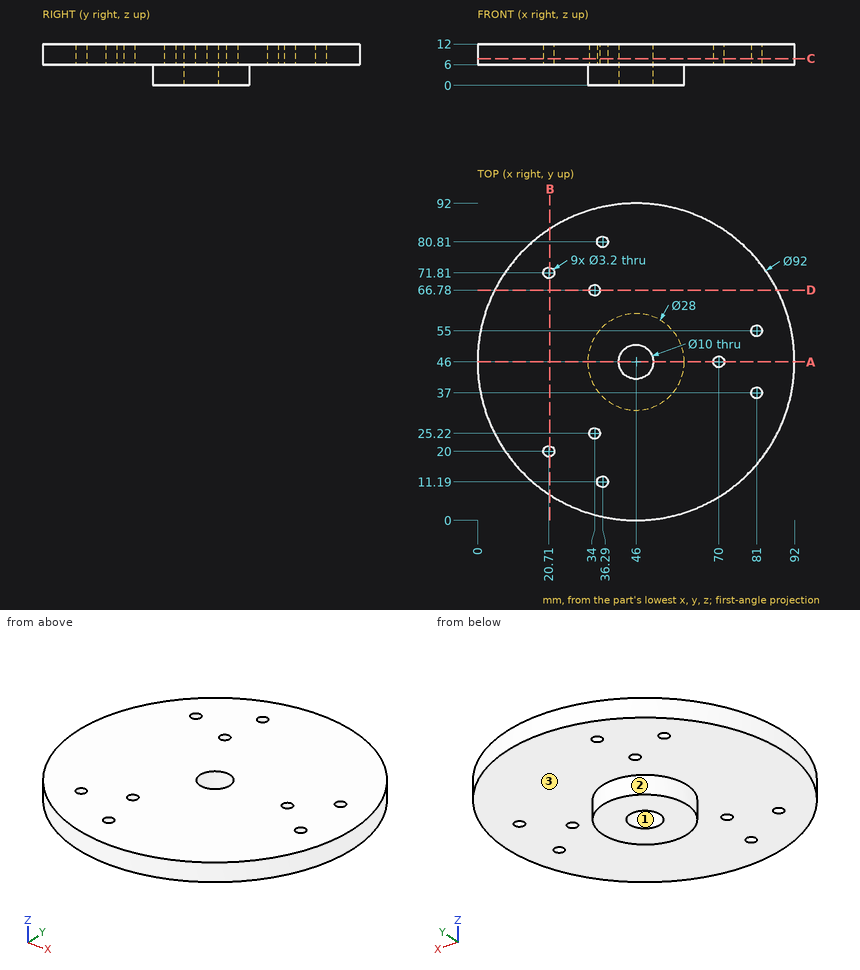
Study the drawing (mm; zero at the part's minimum x, y, z) and answer. Coordinates: 2 decimals unless noted, no trailing zeros. Write each loop counter-clockwise with the first axis right and the second up, starting at its lowest first coordinate (ties: lowest second). Pieces come first, ordered by that corner, then holes.
Q1. Find the intervals of material crossed by line 1 along Y through (x, z) = (36.29, 9.95); line 2 along Y through (x, z) = (81, 7.2); line 3 along Z through (x, y) = (45.5, 20.5), in increasing order.
Returned:
line 1: y = 1.04 to 9.59, 12.79 to 79.21, 82.41 to 90.96
line 2: y = 16.15 to 35.4, 38.6 to 53.4, 56.6 to 75.85
line 3: z = 6 to 12
Q2. Section D-D, the plane y = 66.78 is taken. Write down the section's boundary in (x, z).
Returned:
outline: (4.96, 6) - (32.4, 6) - (32.4, 12) - (4.96, 12) - close; (35.6, 6) - (87.04, 6) - (87.04, 12) - (35.6, 12) - close
Q3. Section B-B, the plane x = 21 is taken. Write down the section's boundary in (y, z).
Returned:
outline: (7.39, 6) - (18.43, 6) - (18.43, 12) - (7.39, 12) - close; (21.57, 6) - (70.24, 6) - (70.24, 12) - (21.57, 12) - close; (73.38, 6) - (84.61, 6) - (84.61, 12) - (73.38, 12) - close
Q4. Section A-A, the plane y = 46 is taken. Write down the section's boundary in (x, z), then the cut area to 3 significant figures.
Returned:
outline: (0, 6) - (32, 6) - (32, 0) - (41, 0) - (41, 12) - (0, 12) - close; (51, 0) - (60, 0) - (60, 6) - (68.4, 6) - (68.4, 12) - (51, 12) - close; (71.6, 6) - (92, 6) - (92, 12) - (71.6, 12) - close
area: 581 mm2
Q5. Given P1, Ø10, axis at x = 34, y = 25.5, coming from the -Z side; P2, Ø4, axis at x = 36.29, y = 80.81, coming from the +Z side; P3, Ø6, axis at x = 48, z = 4.5, coming from the -Y side, each flat-ended and moving along its own axis, determine where each tip first touches the part or whether it passes through.
Returned:
P1: stops at z = 6
P2: stops at z = 12
P3: stops at y = 0
Q6. Section C-C, the plane z = 7.75 is taken. Give the number of separate pieces and of enclosed holes in the cut face, then the cut area to 3 significant figures.
Returned:
separate pieces: 1
enclosed holes: 10
area: 6,500 mm2
Q7. The mould has two halves that part along X. Classify the marked faces 1, 2 and 3: released by +X, released by -X, zero draft, split by the parting line, or undercut.
Returned:
face 1: undercut
face 2: split by the parting line
face 3: zero draft
